Print and shaded views of the part. All mm, measured from the part's lowest x, y and z. A direction names the side the tool comes from. Round coordinates to 2 decimals unless told otherwise and drop trailing zeros. Order: outer loops, then holes, each group sorted by start corner. A loop starts at its lowest first (then second) coordinate and runs counter-clockwise, first axis right, second up. Notation, with made-up numbers: M -34,57 L 23,57 A17 cw 23,65 Z; hole C -14.75,9.5 d10. An arc over 180 degrees is marked long. Use CSV: the item, a comma, the result in double quotes.
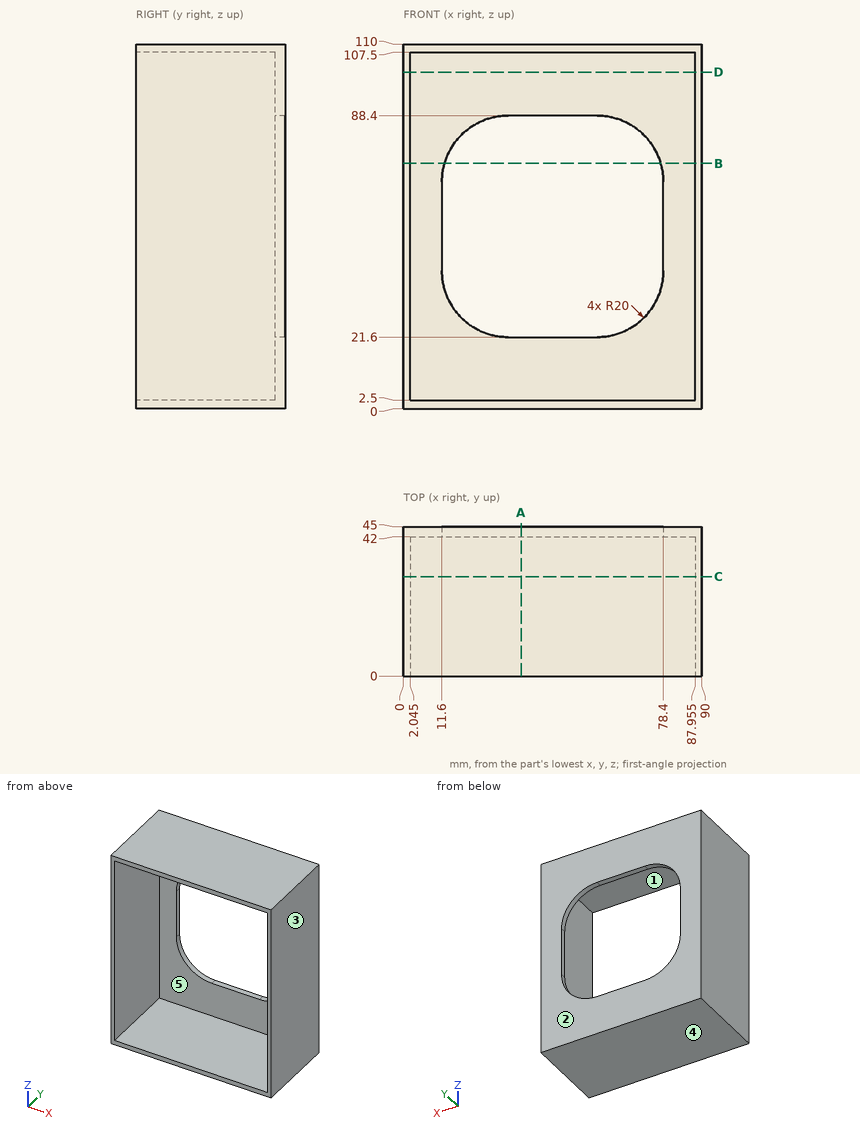
(1) Wall check: line 1 (Z direction, x = 43, y = 9.5); line 2 (X direction, y = 35, z = 49.5) (1 decimal); line 3 (Y direction, x = 8, z = 81). Give the ranges that are in metal, low to high. Write a range as from..to.
Answer block:
line 1,"z = 0..2.5, 107.5..110"
line 2,"x = 0..2, 88..90"
line 3,"y = 42..45"
(2) Tool access for the marked faces 1 and 2: list every direction of +Z, -Z, +X, -X, +Y, -Y with a clear straight run to the whole face (end or side of a thin tool).
Answer block:
face 1,"-Y"
face 2,"+Z, -Z, +X, -X, +Y"
(3) Cut at A-A, the plane x = 35.5. Give the cut face in (y, z).
Answer block:
outline,"M 0,0 L 45,0 L 45,21.6 L 42,21.6 L 42,2.5 L 0,2.5 Z; M 0,107.5 L 42,107.5 L 42,88.4 L 45,88.4 L 45,110 L 0,110 Z"
(4) Drop flat-ended pins along their axis: pin 1 (3.5 mm diameter, centred on y = 44, z = 55.5, fed in from -X); pin 2 (8 mm diameter, centred on x = 73.5, z = 52, fed in from +Y). Give the stop position or say it passes through.
Answer block:
pin 1,"stops at x = 0"
pin 2,"passes through"
(5) Cut at B-B, the plane z = 74. Give the cut face in (x, y) (1 decimal), and give its area (3 significant figures).
Answer block:
outline,"M 0,0 L 2,0 L 2,42 L 12.4,42 L 12.4,45 L 0,45 Z; M 77.6,42 L 88,42 L 88,0 L 90,0 L 90,45 L 77.6,45 Z"
area,"246 mm²"
(6) Cut at C-C, the plane y = 30. Give the cut face in (x, z) (1 decimal).
Answer block:
outline,"M 0,0 L 90,0 L 90,110 L 0,110 Z; hole M 2,2.5 L 88,2.5 L 88,107.5 L 2,107.5 Z"
(7) Two-plate mould, pull along Z, no slides. Class the marked faces 3, 4 and 5: released by +Z, released by -Z, zero draft, split by the parting line, or undercut.
Answer block:
face 3,"zero draft"
face 4,"released by -Z"
face 5,"undercut"
(8) Cut at D-D, the plane z = 101.5. Give the cut face in (x, y) (1 decimal).
Answer block:
outline,"M 0,0 L 2,0 L 2,42 L 88,42 L 88,0 L 90,0 L 90,45 L 0,45 Z"
